Part model, mm, in its own coordinate system. A direction names the side the tool comes from. Coordinates: 2 decimals unless noted, no trailing zeros. Write each loop counter-clockwise with the first axis right and the second up, starting at its lowest first coordinate (ties: lowest second). Pieces come first, ordered by that corner, then holes. Notation, with made-up numbers: (-39, -26.5) -> (-28, -26.5) arc R26 cw to (-28, -3.5) -> close; hole circle Ø4 at (75.25, 47). An arc over 180 degrees is marked (long way). Write item = value, one per line.
Autodesk Inventor part; units mm, degrees
ref_plane "YZ Plane" through (0, 0, 0) normal (1, 0, 0) x (0, 1, 0)
ref_plane "XZ Plane" through (0, 0, 0) normal (0, 1, 0) x (-1, 0, 0)
ref_plane "XY Plane" through (0, 0, 0) normal (0, 0, 1) x (1, 0, 0)
sketch "Sketch1" plane through (0, 0, 0) normal (0, 1, 0) x (-1, 0, 0)
  circle A0 centre (0, 0) radius 19.05
  circle A1 centre (0, 0) radius 41.275 construction
  line L0 (0, -57.15) -> (0, 57.15) construction
  circle A2 centre (0, -57.15) radius 7.9375
  line L1 (57.785, 0) -> (-57.785, 0) construction
  circle A3 centre (0, -57.15) radius 19.05 construction
  circle A4 centre (0, 57.15) radius 7.9375
  circle A5 centre (0, 57.15) radius 19.05 construction
  line L2 (-17.5505, -64.5583) -> (-38.026, -16.0514)
  line L3 (17.5505, -64.5583) -> (38.026, -16.0514)
  line L4 (-17.5505, 64.5583) -> (-38.026, 16.0514)
  line L5 (17.5505, 64.5583) -> (38.026, 16.0514)
  arc A6 (-17.5505, -64.5583) -> (17.5505, -64.5583) centre (0, -57.15) ccw
  arc A7 (17.5505, 64.5583) -> (-17.5505, 64.5583) centre (0, 57.15) ccw
  arc A8 (-38.026, 16.0514) -> (-38.026, -16.0514) centre (0, 0) ccw
  arc A9 (38.026, -16.0514) -> (38.026, 16.0514) centre (0, 0) ccw
  dimension "d1" = 82.55
  dimension "d4" = 38.1
  dimension "d0" = 38.1
  dimension "d2" = 114.3
  dimension "d3" = 15.875
extrude "Extrusion1" add sketch "Sketch1" along normal blind 12.7
sketch "Sketch2" plane through (0, 0, 0) normal (1, 0, 0) x (0, 1, 0)
  line L0 (0, -19.05) -> (12.7, -19.05) construction
  line L1 (12.7, -19.05) -> (19.05, -19.05)
  line L2 (19.05, -19.05) -> (25.4, -12.7)
  line L3 (25.4, -12.7) -> (41.148, -12.7)
  line L4 (41.148, -12.7) -> (41.148, -22.225)
  line L5 (41.148, -22.225) -> (50.8, -22.225)
  line L6 (50.8, -22.225) -> (50.8, -31.0661)
  line L7 (50.8, -31.0661) -> (12.7, -41.275)
  line L8 (12.7, -64.5583) -> (12.7, -16.0514) construction
  line L9 (0, -16.0514) -> (0, -64.5583) construction
  line L10 (12.7, -19.05) -> (12.7, -41.275)
  line L11 (12.7, -19.05) -> (12.7, -41.275)
  line L12 (12.7, -41.275) -> (50.8, -31.0661)
  line L13 (50.8, -31.0661) -> (50.8, -22.225)
  line L14 (41.148, -22.225) -> (50.8, -22.225)
  line L15 (41.148, -22.225) -> (41.148, -12.7)
  line L16 (41.148, -12.7) -> (25.4, -12.7)
  line L17 (25.4, -12.7) -> (19.05, -19.05)
  line L18 (19.05, -19.05) -> (12.7, -19.05)
  line L19 (12.7, -41.275) -> (28.7707, -41.275) construction
  line L20 (-10.16, 0) -> (60.96, 0) construction
  point P0 (0, 0)
  dimension "d7" = 50.8
  dimension "d8" = 19.05
  dimension "d9" = 12.7
  dimension "d10" = 41.275
  dimension "d12" = 22.225
  dimension "d13" = 9.652
  dimension "d14" = 25.4
  dimension "d16" = 15
revolve "Revolution1" add sketch "Sketch2" angle 360 about axis through (0, -10, 0) along (0, 1, 0)
properties part number "SólidoC"
Q1. Probe line 1 (Z direction, x = 0, y = 9); line 2 (Y direction, x = -6, z = -47.5); line 3 (Z direction, x = 0, y = 46) (3 decimals). List the from-to ranges inside material, lowest first. Write a range as from..to.
Model answer:
line_1 = -76.2..-65.09, -49.21..-19.05, 19.05..49.21, 65.09..76.2
line_2 = 0..12.7
line_3 = -32.352..-22.225, 22.225..32.352
Q2. Which spindle directions (+Z, -Z, +X, -X, +Y, -Y) get a long thin tool onto all of the face, cutting with end or side? Do faces 1 (the face through (-6.676, 46.042, -21.199)), 2 (the face through (41.274, 6.261, -0.231)). Say none if no direction does.
Model answer:
face_1 = +Y
face_2 = +X, +Y, -Y
Q3. Pin check, flat tips, straight feed: pin 1 (2 mm diameter, centred on x = -6.5, z = 19, fed in from -Y); pin 2 (1 mm diameter, centred on x = -6, y = 19, fed in from +Z); pin 3 (12 mm diameter, centred on x = 9, y = 44.5, fed in from +Z); pin 4 (1 mm diameter, centred on x = -19.5, y = 28, fed in from +Z). Stop position of each tip, or through.
Model answer:
pin_1 = 0
pin_2 = 39.28
pin_3 = 33.62
pin_4 = 31.99
Q4. Saw through at C-C on z = -57.15. Give the cut face in (x, y), and give its area (3 significant figures).
Model answer:
outline = (-20.68, 0) -> (-7.94, 0) -> (-7.94, 12.7) -> (-20.68, 12.7) -> close; (7.94, 0) -> (20.68, 0) -> (20.68, 12.7) -> (7.94, 12.7) -> close
area = 324 mm²
Q5. Mould opens along Z. For faces 3 (the face through (27.645, 6.261, 40.644)), 4 (the face through (-21.15, 50.8, 7.34)), 5 (the face through (12.4, 33.38, 2.75)) say: released by +Z, released by -Z, zero draft, split by the parting line, or undercut.
Model answer:
face_3 = released by +Z
face_4 = zero draft
face_5 = undercut
Q6. Saw through at B-B on z = 0. Give the cut face in (x, y) (3 decimals).
Model answer:
outline = (-41.275, 0) -> (-19.05, 0) -> (-19.05, 19.05) -> (-12.7, 25.4) -> (-12.7, 41.148) -> (-22.225, 41.148) -> (-22.225, 50.8) -> (-31.066, 50.8) -> (-41.275, 12.7) -> close; (12.7, 25.4) -> (19.05, 19.05) -> (19.05, 0) -> (41.275, 0) -> (41.275, 12.7) -> (31.066, 50.8) -> (22.225, 50.8) -> (22.225, 41.148) -> (12.7, 41.148) -> close
Q7. Saw through at A-A on x = 0. Count the separate pieces of the cut face and the enclosed holes in it, and give its area (3 significant figures).
Model answer:
separate_pieces = 4
enclosed_holes = 0
area = 2,530 mm²
Q8. Saw through at D-D on y = 17. Give the cut face in (x, z), and give its area (3 significant figures).
Model answer:
outline = circle Ø80.25 at (0, 0); hole circle Ø38.1 at (0, 0)
area = 3,920 mm²
